Verification items for the finished model (mm, model axes). Give positions to 0.01 mm unless a question says otherwise; leave off trailing zeros. Write each loop counter-clockwise with the first axis right and the second up, starting at its lowest first coordinate (ties: lowest second). Pieces come first, ordered by that corner, then holes. Notation, with made-up numbers: (-1.75, 65.25) - (8.25, 65.25) arc R20 cw to (8.25, 87.25) - close; hole circle Ø3 at (64, 87.25). An arc over 180 degrees is marked (long way). Put each result on its own line as item: value.
from build123d import *

# Parameters (mm, degrees)
SKETCH1_W           = 199.39
SKETCH1_H           = 177.8
BOSS_EXTRUDE1_DEPTH = 3.175
CUT_EXTRUDE4_DEPTH  = 134.612812447
SKETCH7_R           = 3.175
CUT_EXTRUDE5_DEPTH  = 134.612812447
SKETCH8_W           = 4.699
SKETCH8_H           = 105.199999912
BOSS_EXTRUDE2_DEPTH = 3.175


with BuildPart() as part:
    # Sketch1 → Boss-Extrude1 (new body)
    with BuildSketch(Plane.XY):
        Rectangle(SKETCH1_W, SKETCH1_H)
    extrude(amount=BOSS_EXTRUDE1_DEPTH)

    # Sketch6 → Cut-Extrude4 (cut, through all)
    with BuildSketch(Plane.XY.offset(3.175)):
        Polygon((99.695, 88.9), (99.695, 19.474999912), (-10.795, 88.9), align=None)
    extrude(amount=-CUT_EXTRUDE4_DEPTH, mode=Mode.SUBTRACT)

    # Sketch7 → Cut-Extrude5 (cut, through all)
    with BuildSketch(Plane.XY.offset(3.175)):
        with Locations((-93.345, 82.55)):
            Circle(SKETCH7_R)
        with Locations((-93.345, 9.949999912)):
            Circle(SKETCH7_R)
        with Locations((93.345, 9.949999912)):
            Circle(SKETCH7_R)
        with Locations((-66.675, 9.949999912)):
            Circle(SKETCH7_R)
        with Locations((-41.275, 9.949999912)):
            Circle(SKETCH7_R)
        with Locations((-15.875, 9.949999912)):
            Circle(SKETCH7_R)
        with Locations((9.525, 9.949999912)):
            Circle(SKETCH7_R)
        with Locations((34.925, 9.949999912)):
            Circle(SKETCH7_R)
        with Locations((60.325, 9.949999912)):
            Circle(SKETCH7_R)
        with Locations((-17.145, 82.55)):
            Circle(SKETCH7_R)
        with Locations((-66.675, -82.55)):
            Circle(SKETCH7_R)
        with Locations((-41.275, -82.55)):
            Circle(SKETCH7_R)
        with Locations((-15.875, -82.55)):
            Circle(SKETCH7_R)
        with Locations((9.525, -82.55)):
            Circle(SKETCH7_R)
        with Locations((34.925, -82.55)):
            Circle(SKETCH7_R)
        with Locations((60.325, -82.55)):
            Circle(SKETCH7_R)
    extrude(amount=-CUT_EXTRUDE5_DEPTH, mode=Mode.SUBTRACT)

    # Sketch8 → Boss-Extrude2 (add)
    with BuildSketch(Plane.XY.offset(3.175)):
        with Locations((-80.137, -36.300000044)):
            Rectangle(SKETCH8_W, SKETCH8_H)
        with Locations((73.787, -36.300000044)):
            Rectangle(SKETCH8_W, SKETCH8_H)
    extrude(amount=BOSS_EXTRUDE2_DEPTH)


solid = part.part
Q1. Release check for a two-part mould opening along Y. For faces 1 (the face through (45.223, 53.702, 1.61)), 2 (the face through (-1, 1, 0)), 3 (the face through (-43.615, -80.404, 1.61)) record: released by +Y, released by -Y, zero draft, split by the parting line, or undercut.
Answers follow:
face 1: released by +Y
face 2: zero draft
face 3: undercut
Q2. Scan lines: line 1 along Z through (x, y) = (-21.5, -4.5) (3 decimals); line 2 along Y through (x, z) = (-18, 1.25); line 3 along X through (y, z) = (-7, 5.25). Record each from-to range of solid material in increasing order.
Answers follow:
line 1: z = 0 to 3.175
line 2: y = -88.9 to -84.91, -80.19 to 7.59, 12.31 to 79.49, 85.61 to 88.9
line 3: x = -82.49 to -77.79, 71.44 to 76.14
Q3. Section check B-B, the plane y = 82.55. Record the cut outline in (x, z) (3 decimals), plus the area to 3 significant figures.
Answers follow:
outline: (-99.695, 0) - (-96.52, 0) - (-96.52, 3.175) - (-99.695, 3.175) - close; (-90.17, 0) - (-20.32, 0) - (-20.32, 3.175) - (-90.17, 3.175) - close; (-13.97, 0) - (-0.689, 0) - (-0.689, 3.175) - (-13.97, 3.175) - close
area: 274 mm2
Q4. Go/stop test with flat-tipped pins: pin 1 Ø4 at (x, y) = (-23, 33) entering from +Z (3 decimals); pin 2 Ø2.5 at (x, z) = (73, 5) entering from +Y; pin 3 Ø1 at (y, z) = (-11, 5.5) entering from -X. Record where each tip stops, or that it passes through.
Answers follow:
pin 1: stops at z = 3.175
pin 2: stops at y = 16.3
pin 3: stops at x = -82.49
Q5. Section check A-A, the plane z = 1.5. Give the number of separate pieces and of enclosed holes in the cut face, plus the area to 3 significant figures.
Answers follow:
separate pieces: 1
enclosed holes: 16
area: 31,100 mm2
